Verification items for the finished model (mm, model axes). Give positions to 0.01 mm unless a question says otherwise; leave off trailing zeros.
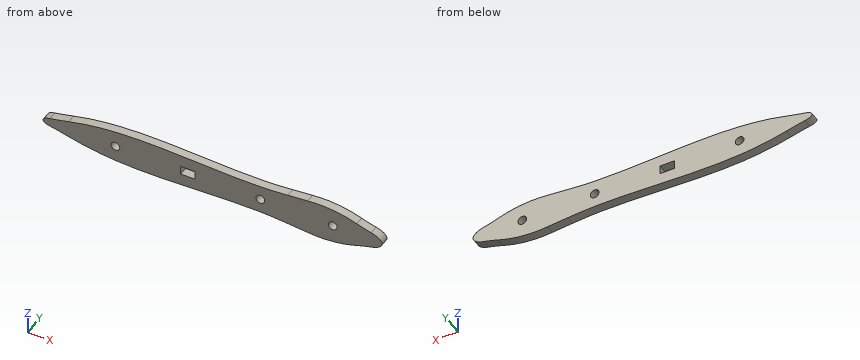
from build123d import *

# Parameters (mm, degrees)
ESBO_O1_R                = 1.5
ESBO_O1_W                = 5
ESBO_O1_H                = 3
RESSALTO_EXTRUS_O1_DEPTH = 3


with BuildPart() as part:
    # Esboço1 → Ressalto-extrusão1 (new body)
    with BuildSketch(Plane(origin=(0, 0, 0), x_dir=(1, 0, 0), z_dir=(0, 1, 0))):
        with BuildLine():
            Line((-15.5324261, 5.526900759), (-8.701477822, 6.15))
            add(Edge.make_bspline(
                [(8.269723742, 4.259468977), (2.834912713, 6.157347241), (-2.82215339, 6.787527354), (-8.701477822, 6.15)],
                knots=[0.35388944, 0.35388944, 0.35388944, 0.35388944, 1, 1, 1, 1], degree=3))
            ThreePointArc((8.269723742, 4.259468977), (10.737611567, 3.46879666), (13.24315076, 2.807051708))
            add(Edge.make_bspline(
                [(13.243153259, -2.80704963), (25.10877849, 2.12e-06), (13.24315076, 2.807051708)],
                knots=[5.194112275, 5.194112275, 5.194112275, 7.372258742, 7.372258742, 7.372258742], degree=2, weights=[1, 0.463306864, 1]))
            ThreePointArc((13.243153259, -2.80704963), (10.737612779, -3.468795552), (8.269723742, -4.259468977))
            add(Edge.make_bspline(
                [(8.269723742, -4.259468977), (2.834913243, -6.15734876), (-2.822153925, -6.787525817), (-8.701477822, -6.15)],
                knots=[0.35388944, 0.35388944, 0.35388944, 0.35388944, 1, 1, 1, 1], degree=3))
            Line((-8.701477822, -6.15), (-15.5324261, -5.526900759))
            add(Edge.make_bspline(
                [(-91.135478662, -2.939356415), (-85.814709071, -4.330378827), (-60.917561227, -7.97508816), (-35.132432713, -3.48955228), (-15.5324261, -5.526900759)],
                knots=[0.107974898, 0.107974898, 0.107974898, 0.107974898, 0.300967181, 1, 1, 1, 1], degree=3))
            ThreePointArc((-91.135478662, -2.939356415), (-94.330524557, -2.159963767), (-97.549471293, -1.486054958))
            add(Edge.make_bspline(
                [(-97.549471293, 1.486054958), (-105.279311729, 0), (-97.549471293, -1.486054958)],
                knots=[5.195092838, 5.195092838, 5.195092838, 7.371277776, 7.371277776, 7.371277776], degree=2, weights=[1, 0.464175793, 1]))
            ThreePointArc((-97.549471293, 1.486054958), (-94.330524557, 2.159963767), (-91.135478662, 2.939356415))
            add(Edge.make_bspline(
                [(-91.135478662, 2.939356415), (-85.814709071, 4.330378827), (-60.917561227, 7.97508816), (-35.132432713, 3.48955228), (-15.5324261, 5.526900759)],
                knots=[0.107974898, 0.107974898, 0.107974898, 0.107974898, 0.300967181, 1, 1, 1, 1], degree=3))
        make_face()
        Circle(ESBO_O1_R, mode=Mode.SUBTRACT)
        with Locations((-75, 0)):
            Circle(ESBO_O1_R, mode=Mode.SUBTRACT)
        with Locations((-25, 0)):
            Circle(ESBO_O1_R, mode=Mode.SUBTRACT)
        with Locations((-50, 0)):
            Rectangle(ESBO_O1_W, ESBO_O1_H, mode=Mode.SUBTRACT)
    extrude(amount=RESSALTO_EXTRUS_O1_DEPTH)


solid = part.part
Item 1: Sectioned sample at A-A on y = 0.7. State how many separate pieces and enclosed holes the cut face has, then the cut area to 3 significant figures.
Answer key:
separate pieces: 1
enclosed holes: 4
area: 1,110 mm2
Item 2: Depth check by flat-ended pin: pin 1 (0.9 mm diameter, centred on x = -51, y = 1.5, fed in from +Z); pin 2 (1 mm diameter, centred on y = 0.5, z = -1, fed in from -X); pin 3 (2.5 mm diameter, centred on x = -25, z = 0, fed in from +Y). Enter the tip coordinate at first touch or a pass-through.
Answer key:
pin 1: stops at z = 5.59
pin 2: stops at x = -99.79
pin 3: passes through
Item 3: Scan lines: line 1 along X through (y, z) = (1.65, 0); line 2 along Z through (x, y) = (0, 1.9); line 3 along Z through (x, y) = (-65.5, 2.55). Record each from-to range of solid material in increasing order.
Answer key:
line 1: x = -100 to -76.5, -73.5 to -52.5, -47.5 to -26.5, -23.5 to -1.5, 1.5 to 17
line 2: z = -6.15 to -1.5, 1.5 to 6.15
line 3: z = -5.9 to 5.9
